Autodesk Inventor part; units mm, degrees
ref_plane "YZ Plane" through (0, 0, 0) normal (1, 0, 0) x (0, 1, 0)
ref_plane "XZ Plane" through (0, 0, 0) normal (0, 1, 0) x (-1, 0, 0)
ref_plane "XY Plane" through (0, 0, 0) normal (0, 0, 1) x (1, 0, 0)
sketch "Sketch1" plane through (0, 0, 0) normal (0, 1, 0) x (-1, 0, 0)
  line L0 (200.025, 436.88) -> (-200.025, 436.88)
  line L1 (-200.025, 436.88) -> (-200.025, -436.88)
  line L2 (-200.025, -436.88) -> (200.025, -436.88)
  line L3 (200.025, -436.88) -> (200.025, 436.88)
  line L4 (200.025, 436.88) -> (-200.025, -436.88) construction
  line L5 (-200.025, 436.88) -> (200.025, -436.88) construction
  point P0 (0, 0)
  dimension "d0" = 400.05
  dimension "d1" = 873.76
extrude "Extrusion1" add sketch "Sketch1" along normal blind 12.7
sketch "Sketch4" plane through (0, 12.7, 0) normal (0, 1, 0) x (1, 0, 0)
  line L0 (-82.55, -436.88) -> (82.55, -436.88)
  line L1 (82.55, -436.88) -> (82.55, -233.68)
  line L2 (82.55, -233.68) -> (-82.55, -233.68)
  line L3 (-82.55, -233.68) -> (-82.55, -436.88)
  line L4 (-82.55, -436.88) -> (82.55, -233.68) construction
  line L5 (82.55, -436.88) -> (-82.55, -233.68) construction
  line L6 (-200.025, -436.88) -> (200.025, -436.88)
  line L7 (-200.025, 436.88) -> (-200.025, -436.88)
  line L8 (200.025, -436.88) -> (200.025, 436.88)
  point P0 (0, 0)
  point P1 (0, -335.28)
  dimension "d11" = 0
  dimension "d12" = 165.1
  dimension "d13" = 203.2
  dimension "d19" = 117.475
  dimension "d20" = 117.475
extrude "Extrusion2" cut sketch "Sketch4" against normal through all
sketch "Sketch6" plane through (0, 12.7, 0) normal (0, 1, 0) x (1, 0, 0)
  line L0 (0, 0) -> (0, -436.88) construction
  line L1 (-127, -360.68) -> (127, -360.68)
  line L2 (127, -360.68) -> (127, -436.88)
  line L3 (127, -436.88) -> (-127, -436.88)
  line L4 (-127, -436.88) -> (-127, -360.68)
  line L5 (-127, -360.68) -> (127, -436.88) construction
  line L6 (127, -360.68) -> (-127, -436.88) construction
  line L7 (-200.025, -436.88) -> (-82.55, -436.88)
  point P0 (0, -398.78)
  dimension "d24" = 254
  dimension "d25" = 76.2
extrude "Extrusion4" cut sketch "Sketch6" against normal through all
properties part number "2020 Wood Base" material "Wood (Birch)"
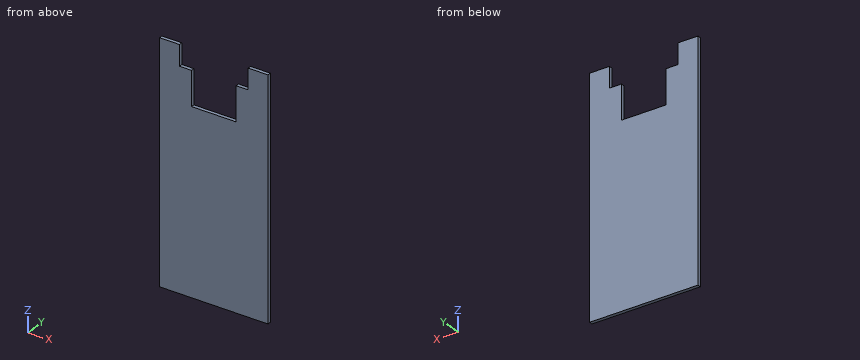
CAD build for the part. Positions are in the model's coordinates, mm. Give positions to 0.01 mm unless a question says otherwise; leave off trailing zeros. Write each loop counter-clockwise with the first axis right and the second up, starting at its lowest first coordinate (ties: lowest second). Pieces come first, ordered by that corner, then holes. Notation, with made-up numbers: M -38,-27.75 L 5,-27.75 A31 ccw 5,3.25 Z; hole C 42.5,85 d10. An arc over 180 degrees is marked long. Return JSON: item names as keys, results as strings. Group by question number.
(1) Band-saw the part on A-A (z = 269). Give the cut face in (x, y) (3 decimals).
(2) Band-saw the part on B-B (y = 6). Give the cut face in (x, z) (3 decimals).
(3) Drill centre lines: L1, parallel to X at y = 6.5, z = 313 (3 decimals); L2, parallel to Z at x = 93, y = 9; L3, parallel to Z at x = -4.5, y = 4.75. Where is each one in solid material? Low to high. Write a range as [from, to].
(4) Band-saw the part on C-C (x = 91.5). Give the cut face in (y, z).
(5) Band-saw the part on D-D (x = 6). Give the cut face in (y, z), and give its area (3 significant figures).
(6) Flat gauge pins, fed straight in: pin 1 Ø3 at (x, y) = (19.5, 4) entering from +Z; pin 2 Ø6.5 at (x, y) = (114, 6.5) entering from +Z; pin 3 Ø1 at (x, z) = (49, 206.5) entering from -Y. Where does each tip first touch, or does it go through?
Entries:
{
 "1": {"outline": "M -200.025,0 L -82.55,0 L -82.55,12.7 L -200.025,12.7 Z; M 82.55,0 L 200.025,0 L 200.025,12.7 L 82.55,12.7 Z"},
 "2": {"outline": "M -200.025,-436.88 L 200.025,-436.88 L 200.025,436.88 L 127,436.88 L 127,360.68 L 82.55,360.68 L 82.55,233.68 L -82.55,233.68 L -82.55,360.68 L -127,360.68 L -127,436.88 L -200.025,436.88 Z"},
 "3": {"L1": "x = [-200.025, -82.55], [82.55, 200.025]", "L2": "z = [-436.88, 360.68]", "L3": "z = [-436.88, 233.68]"},
 "4": {"outline": "M 0,-436.88 L 12.7,-436.88 L 12.7,360.68 L 0,360.68 Z"},
 "5": {"outline": "M 0,-436.88 L 12.7,-436.88 L 12.7,233.68 L 0,233.68 Z", "area": "8,520 mm^2"},
 "6": {"pin 1": "stops at z = 233.68", "pin 2": "stops at z = 360.68", "pin 3": "stops at y = 0"}
}
